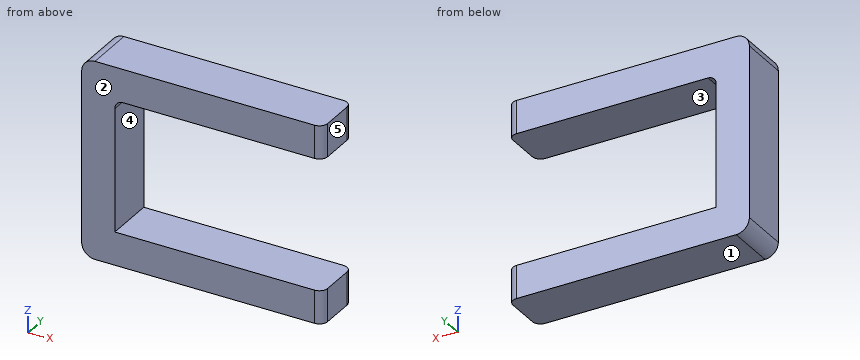
```python
from build123d import *

# Parameters (mm, degrees)
EXTRUDE4_DEPTH       = 38.1
FILLET1_R            = 6.35
FILLET2_R            = 10.16
FILLET2_OF_MIRROR1_R = 10.16
FILLET4_R            = 6.35


with BuildPart() as part:
    # Sketch4 → Extrude4 (new body)
    with BuildSketch(Plane(origin=(0, 0, 0), x_dir=(1, 0, 0), z_dir=(0, 1, 0))):
        Polygon((-25.4, -25.4), (159.67622317, -25.4), (159.67622317, 0), (0, 0), (0, 50.356184866), (-25.4, 50.356184866), align=None)
    extrude4 = extrude(amount=-EXTRUDE4_DEPTH)

    # Fillet1
    fillet1_edges = [part.edges().sort_by_distance(p)[0] for p in [
        (0, -19.05, 0),
        (159.67622317, -38.1, 12.7),
        (159.67622317, 0, 12.7),
    ]]
    fillet(fillet1_edges, radius=FILLET1_R)

    # Fillet2
    fillet2_edges = [part.edges().sort_by_distance(p)[0] for p in [
        (-25.4, -19.05, 25.4),
    ]]
    fillet(fillet2_edges, radius=FILLET2_R)

    # Mirror1: Extrude4 across plane
    add(extrude4.mirror(Plane(origin=(-25.4, -38.1, -50.356184866), x_dir=(1, 0, 0), z_dir=(0, 0, -1))))

    # Fillet2 of Mirror1
    fillet2_of_mirror1_edges = [part.edges().sort_by_distance(p)[0] for p in [
        (-25.4, -19.05, -126.112369731),
    ]]
    fillet(fillet2_of_mirror1_edges, radius=FILLET2_OF_MIRROR1_R)

    # Fillet4
    fillet4_edges = [part.edges().sort_by_distance(p)[0] for p in [
        (159.67622317, 0, -113.412369731),
        (159.67622317, -38.1, -113.412369731),
    ]]
    fillet(fillet4_edges, radius=FILLET4_R)


solid = part.part
```
Check sheet for the modelled part. Datum: model origin and axes. Units: mm. Face numbers are marked on the shaded views. A direction names the side the tool comes from. Coordinates: 2 decimals unless noted, no trailing zeros. Loops run counter-clockwise (first coordinate to the right, second up) from the corner with the lowest first, then second, coordinate; pieces in that order, holes last. Notation, with made-up numbers: M 58,-31.75 L 69,-31.75 A9 cw 69,-16.75 Z; hole C 74,23.5 d1. An arc over 180 degrees is marked long. Answer as a JSON object with one key per item and string values.
1. Sectioned sample at D-D on y = -35. Record the cut outline in (x, z), and give its area (3 significant figures).
Outcome:
{"outline": "M -25.4,-115.95 A10.16 ccw -15.24,-126.11 L 158.78,-126.11 L 158.78,-100.71 L 0,-100.71 L 0,-6.35 A6.35 cw 6.35,0 L 158.78,0 L 158.78,25.4 L -15.24,25.4 A10.16 ccw -25.4,15.24 Z", "area": "11,900 mm²"}
2. Sectioned sample at A-A on x = 83. Record the cut outline in (y, z).
Outcome:
{"outline": "M -38.1,-126.11 L 0,-126.11 L 0,-100.71 L -38.1,-100.71 Z; M -38.1,0 L 0,0 L 0,25.4 L -38.1,25.4 Z"}
3. Depth check by flat-ended pin: P1, Ø2, axis at y = -24.5, z = -43.5, coming from the +X side. Enter the tip coordinate at first touch or a pass-through.
Outcome:
{"P1": "x = 0"}
4. Sectioned sample at C-C on z = -77.5. Record the cut outline in (x, y), and give its area (3 significant figures).
Outcome:
{"outline": "M -25.4,-38.1 L 0,-38.1 L 0,0 L -25.4,0 Z", "area": "968 mm²"}
5. Release check for a two-part mould opening along Z. For the marked faces 1, 2 and 3 record: pulls with the +Z half, pulls with the -Z half, needs draft (parallel to the pull), parting line crosses it, or undercut.
Outcome:
{"face 1": "pulls with the -Z half", "face 2": "needs draft", "face 3": "undercut"}
6. Scan lines: L1, parallel to Z at x = 146.5, y = -19; L2, parallel to X at y = -30, z = -78; L3, parallel to Z at x = 5, y = -14.5. Record each from-to range of solid material in increasing order. Write a range as from..to.
Outcome:
{"L1": "-126.11..-100.71, 0..25.4", "L2": "-25.4..0", "L3": "-126.11..-100.71, -0.15..25.4"}
7. Access from +Z, -Z, +X, -X, +Y, -Y to the whole of each face (thin tool, end or side, straight path). Record for the marked faces 4 and 5.
Outcome:
{"face 4": "+X, +Y, -Y", "face 5": "+Z, -Z, +X, +Y, -Y"}
8. Sectioned sample at B-B on y = -24. Record the cut outline in (x, z), and give its area (3 significant figures).
Outcome:
{"outline": "M -25.4,-115.95 A10.16 ccw -15.24,-126.11 L 159.68,-126.11 L 159.68,-100.71 L 0,-100.71 L 0,-6.35 A6.35 cw 6.35,0 L 159.68,0 L 159.68,25.4 L -15.24,25.4 A10.16 ccw -25.4,15.24 Z", "area": "11,900 mm²"}
